The listing builds one solid part. Answer for the finished solid, in the listing's coordinates (mm). A direction names the side the tool comes from. Give positions to 0.01 mm unless a question says otherwise; leave off trailing zeros. Write each loop counter-clockwise with the first axis right and the second up, starting at its lowest first coordinate (ties: lowest second). Pieces come first, ordered by that corner, then holes. Notation, with made-up numbers: (20.5, 12.25) - (61.5, 12.25) arc R12 cw to (61.5, 27.25) - close; hole circle Ø4 at (67, -8). An arc over 180 degrees is marked (long way). Write each question's results on one line, items separated by ' | '. Start each with the question number.
Q1. For a pull along Y with two mould halves and no side action, classify faces 4 (the face through (-1, -15, 1)), 5 (the face through (-0.9, 16, -34.7)), 6 (the face through (-34.068, 5.088, -54.986)) as pulls with the +Y half, pulls with the -Y half, needs draft (parallel to the pull), parting line crosses it, or undercut.
Q2. Section C-C (y = 0) is taken. Determine the outline of the cut face in (x, z).
Q3. For faces 1 (the face through (-1, -15, -55)), 2 (the face through (-34.068, -4.912, -54.986)), 3 (the face through (-1, 0, -54)), determine the directions among +Z, -Z, +X, -X, +Y, -Y from which every point of the face is accessible in a straight line to the end or side of a thin tool.
Q4. Section B-B (x = 17.42) is taken. Determine the outline of the cut face in (y, z).
Q5. Flat-ended cylindrical pins translate along their axes: pin 1 Ø5 at (x, y) = (17, 0) entering from +Z; pin 2 Ø3.5 at (x, z) = (-6.5, -27) entering from -Y; pin 3 Ø16 at (x, y) = (-17, 0) entering from -Z. Find the tip coordinate at first contact, or state that the pin passes through.
Q6. Section A-A (x = -23) is taken. Determine the outline of the cut face in (y, z).
Q7. Find the intervals of material crossed by probe 1 along Y at (x, z) = (-32.07, -55.55); probe 2 along Z at (x, y) = (0, -6); probe 3 along Y at (x, z) = (-18.5, -17), in increasing order.
Q8. Section D-D (z = -33.5) is taken. Determine the outline of the cut face in (x, y), plus the area to 3 significant figures.
```python
from build123d import *

# Parameters (mm, degrees)
SKETCH_1_W          = 80
SKETCH_1_H          = 30
EXTRUDE_1_DEPTH     = 2
SKETCH_2_W          = 80
SKETCH_2_H          = 58
EXTRUDE_2_DEPTH     = 2
SKETCH_3_W          = 80
SKETCH_3_H          = 2
EXTRUDE_3_DEPTH     = 30
CUT_EXTRUDE_1_REACH = 77.895
SKETCH_5_R          = 4.5
SKETCH_5_R_2        = 1.5
CUT_EXTRUDE_3_REACH = 74.478
SKETCH_6_R          = 1.5
CUT_EXTRUDE_4_REACH = 74.478
SKETCH_7_R          = 10
CUT_EXTRUDE_5_REACH = 72.887
SKETCH_8_R          = 2
CUT_EXTRUDE_6_REACH = 72.887
SKETCH_9_R          = 2


with BuildPart() as part:
    # 草图1 → 凸台-拉伸1 (new body)
    with BuildSketch(Plane.XY):
        Rectangle(SKETCH_1_W, SKETCH_1_H)
    extrude(amount=EXTRUDE_1_DEPTH)

    # 草图2 → 凸台-拉伸2 (add)
    with BuildSketch(Plane(origin=(0, 15, 0), x_dir=(1, 0, 0), z_dir=(0, 1, 0))):
        with Locations((0, 27)):
            Rectangle(SKETCH_2_W, SKETCH_2_H)
    extrude(amount=EXTRUDE_2_DEPTH)

    # 草图3 → 凸台-拉伸3 (add)
    with BuildSketch(Plane.XZ.offset(-15)):
        with Locations((0, -55)):
            Rectangle(SKETCH_3_W, SKETCH_3_H)
    extrude(amount=EXTRUDE_3_DEPTH)

    # 草图5 → 切除-拉伸1 (cut, up to next)
    with BuildSketch(Plane(origin=(0, 17, 0), x_dir=(1, 0, 0), z_dir=(0, 1, 0)), mode=Mode.PRIVATE) as cut_extrude_1_sk1:
        with Locations(Location((0, 27, 0), (0, 0, 270))):
            Circle(SKETCH_5_R)
    cut_extrude_1_tool1 = extrude(cut_extrude_1_sk1.sketch, amount=-CUT_EXTRUDE_1_REACH, mode=Mode.PRIVATE) & part.part
    # 草图5 → 切除-拉伸1 (cut, up to next)
    with BuildSketch(Plane(origin=(0, 17, 0), x_dir=(1, 0, 0), z_dir=(0, 1, 0)), mode=Mode.PRIVATE) as cut_extrude_1_sk2:
        with Locations(Location((-6.5, 27, 0), (0, 0, 270))):
            Circle(SKETCH_5_R_2)
    cut_extrude_1_tool2 = extrude(cut_extrude_1_sk2.sketch, amount=-CUT_EXTRUDE_1_REACH, mode=Mode.PRIVATE) & part.part
    # 草图5 → 切除-拉伸1 (cut, up to next)
    with BuildSketch(Plane(origin=(0, 17, 0), x_dir=(1, 0, 0), z_dir=(0, 1, 0)), mode=Mode.PRIVATE) as cut_extrude_1_sk3:
        with Locations(Location((6.5, 27, 0), (0, 0, 270))):
            Circle(SKETCH_5_R_2)
    cut_extrude_1_tool3 = extrude(cut_extrude_1_sk3.sketch, amount=-CUT_EXTRUDE_1_REACH, mode=Mode.PRIVATE) & part.part
    # 草图5 → 切除-拉伸1 (cut, up to next)
    with BuildSketch(Plane(origin=(0, 17, 0), x_dir=(1, 0, 0), z_dir=(0, 1, 0)), mode=Mode.PRIVATE) as cut_extrude_1_sk4:
        with Locations(Location((0, 33.5, 0), (0, 0, 270))):
            Circle(SKETCH_5_R_2)
    cut_extrude_1_tool4 = extrude(cut_extrude_1_sk4.sketch, amount=-CUT_EXTRUDE_1_REACH, mode=Mode.PRIVATE) & part.part
    # 草图5 → 切除-拉伸1 (cut, up to next)
    with BuildSketch(Plane(origin=(0, 17, 0), x_dir=(1, 0, 0), z_dir=(0, 1, 0)), mode=Mode.PRIVATE) as cut_extrude_1_sk5:
        with Locations(Location((0, 20.5, 0), (0, 0, 270))):
            Circle(SKETCH_5_R_2)
    cut_extrude_1_tool5 = extrude(cut_extrude_1_sk5.sketch, amount=-CUT_EXTRUDE_1_REACH, mode=Mode.PRIVATE) & part.part
    add(cut_extrude_1_tool1.solids().sort_by_distance((0, 17, -27))[0], mode=Mode.SUBTRACT)
    add(cut_extrude_1_tool2.solids().sort_by_distance((-6.5, 17, -27))[0], mode=Mode.SUBTRACT)
    add(cut_extrude_1_tool3.solids().sort_by_distance((6.5, 17, -27))[0], mode=Mode.SUBTRACT)
    add(cut_extrude_1_tool4.solids().sort_by_distance((0, 17, -33.5))[0], mode=Mode.SUBTRACT)
    add(cut_extrude_1_tool5.solids().sort_by_distance((0, 17, -20.5))[0], mode=Mode.SUBTRACT)

    # 切除-拉伸3: up to this face of the body (flat: up to its plane)
    cut_extrude_3_end = Plane(part.part.faces().sort_by_distance((0, 1, 2))[0])
    # 草图6 → 切除-拉伸3 (cut, up to the picked face)
    with BuildSketch(Plane(origin=(0, 0, -56), x_dir=(-1, 0, 0), z_dir=(0, 0, -1)), mode=Mode.PRIVATE) as cut_extrude_3_sk1:
        with Locations((-17, 0)):
            Circle(SKETCH_6_R)
    cut_extrude_3_tool1 = split(extrude(cut_extrude_3_sk1.sketch, amount=-CUT_EXTRUDE_3_REACH, mode=Mode.PRIVATE), bisect_by=cut_extrude_3_end, keep=Keep.BOTH, mode=Mode.PRIVATE)
    # 草图6 → 切除-拉伸3 (cut, up to the picked face)
    with BuildSketch(Plane(origin=(0, 0, -56), x_dir=(-1, 0, 0), z_dir=(0, 0, -1)), mode=Mode.PRIVATE) as cut_extrude_3_sk2:
        with Locations((17, 0)):
            Circle(SKETCH_6_R)
    cut_extrude_3_tool2 = split(extrude(cut_extrude_3_sk2.sketch, amount=-CUT_EXTRUDE_3_REACH, mode=Mode.PRIVATE), bisect_by=cut_extrude_3_end, keep=Keep.BOTH, mode=Mode.PRIVATE)
    add(cut_extrude_3_tool1.solids().sort_by(Axis((17, 0, -56), (0, 0, 1)))[0], mode=Mode.SUBTRACT)
    add(cut_extrude_3_tool2.solids().sort_by(Axis((-17, 0, -56), (0, 0, 1)))[0], mode=Mode.SUBTRACT)

    # 草图7 → 切除-拉伸4 (cut, up to next)
    with BuildSketch(Plane(origin=(0, 0, -56), x_dir=(-1, 0, 0), z_dir=(0, 0, -1)), mode=Mode.PRIVATE) as cut_extrude_4_sk1:
        with Locations((17, 0)):
            Circle(SKETCH_7_R)
    cut_extrude_4_tool1 = extrude(cut_extrude_4_sk1.sketch, amount=-CUT_EXTRUDE_4_REACH, mode=Mode.PRIVATE) & part.part
    add(cut_extrude_4_tool1.solids().sort_by_distance((-17, 0, -56))[0], mode=Mode.SUBTRACT)

    # 草图8 → 切除-拉伸5 (cut, up to next)
    with BuildSketch(Plane.XY.offset(-54), mode=Mode.PRIVATE) as cut_extrude_5_sk1:
        with Locations((17.42, 5)):
            Circle(SKETCH_8_R)
    cut_extrude_5_tool1 = extrude(cut_extrude_5_sk1.sketch, amount=-CUT_EXTRUDE_5_REACH, mode=Mode.PRIVATE) & part.part
    # 草图8 → 切除-拉伸5 (cut, up to next)
    with BuildSketch(Plane.XY.offset(-54), mode=Mode.PRIVATE) as cut_extrude_5_sk2:
        with Locations((17.42, -5)):
            Circle(SKETCH_8_R)
    cut_extrude_5_tool2 = extrude(cut_extrude_5_sk2.sketch, amount=-CUT_EXTRUDE_5_REACH, mode=Mode.PRIVATE) & part.part
    add(cut_extrude_5_tool1.solids().sort_by_distance((17.42, 5, -54))[0], mode=Mode.SUBTRACT)
    add(cut_extrude_5_tool2.solids().sort_by_distance((17.42, -5, -54))[0], mode=Mode.SUBTRACT)

    # 草图9 → 切除-拉伸6 (cut, up to next)
    with BuildSketch(Plane.XY.offset(-54), mode=Mode.PRIVATE) as cut_extrude_6_sk1:
        with Locations((-32.07, 5)):
            Circle(SKETCH_9_R)
    cut_extrude_6_tool1 = extrude(cut_extrude_6_sk1.sketch, amount=-CUT_EXTRUDE_6_REACH, mode=Mode.PRIVATE) & part.part
    # 草图9 → 切除-拉伸6 (cut, up to next)
    with BuildSketch(Plane.XY.offset(-54), mode=Mode.PRIVATE) as cut_extrude_6_sk2:
        with Locations((-32.07, -5)):
            Circle(SKETCH_9_R)
    cut_extrude_6_tool2 = extrude(cut_extrude_6_sk2.sketch, amount=-CUT_EXTRUDE_6_REACH, mode=Mode.PRIVATE) & part.part
    add(cut_extrude_6_tool1.solids().sort_by_distance((-32.07, 5, -54))[0], mode=Mode.SUBTRACT)
    add(cut_extrude_6_tool2.solids().sort_by_distance((-32.07, -5, -54))[0], mode=Mode.SUBTRACT)


solid = part.part
```
Answers below:
1) face 4: pulls with the -Y half | face 5: needs draft | face 6: undercut
2) outline: (-40, -56) - (-27, -56) - (-27, -54) - (-40, -54) - close; (-40, 0) - (-18.5, 0) - (-18.5, 2) - (-40, 2) - close; (-15.5, 0) - (15.5, 0) - (15.5, 2) - (-15.5, 2) - close; (-7, -56) - (15.5, -56) - (15.5, -54) - (-7, -54) - close; (18.5, -56) - (40, -56) - (40, -54) - (18.5, -54) - close; (18.5, 0) - (40, 0) - (40, 2) - (18.5, 2) - close
3) face 1: +Z, -Z, +X, -X, -Y | face 2: -Z | face 3: +X, -X, -Y
4) outline: (-15, -56) - (-7, -56) - (-7, -54) - (-15, -54) - close; (-15, 0) - (-1.44, 0) - (-1.44, 2) - (-15, 2) - close; (-3, -56) - (-1.44, -56) - (-1.44, -54) - (-3, -54) - close; (1.44, -56) - (3, -56) - (3, -54) - (1.44, -54) - close; (1.44, 0) - (15, 0) - (15, -54) - (7, -54) - (7, -56) - (17, -56) - (17, 2) - (1.44, 2) - close
5) pin 1: stops at z = 2 | pin 2: stops at y = 15 | pin 3: stops at z = 0
6) outline: (-15, -56) - (-8, -56) - (-8, -54) - (-15, -54) - close; (-15, 0) - (15, 0) - (15, -54) - (8, -54) - (8, -56) - (17, -56) - (17, 2) - (-15, 2) - close
7) probe 1: y = -15 to -7, -3 to 3, 7 to 17 | probe 2: z = -56 to -54, 0 to 2 | probe 3: y = 15 to 17
8) outline: (-40, 15) - (-1.5, 15) - (-1.5, 17) - (-40, 17) - close; (1.5, 15) - (40, 15) - (40, 17) - (1.5, 17) - close | area: 154 mm2
